```python
from build123d import *

# Parameters (mm, degrees)
SKETCH_1_W          = 18.46
SKETCH_1_H          = 19.3
EXTRUDE_1_DEPTH     = 1
CUT_EXTRUDE_1_DEPTH = 2


with BuildPart() as part:
    # 草图1 → 凸台-拉伸1 (new body)
    with BuildSketch(Plane(origin=(0, 0, 0), x_dir=(1, 0, 0), z_dir=(0, 1, 0))):
        Rectangle(SKETCH_1_W, SKETCH_1_H)
    extrude(amount=EXTRUDE_1_DEPTH)

    # 草图2 → 切除-拉伸1 (cut, through all)
    with BuildSketch(Plane(origin=(0, 1, 0), x_dir=(1, 0, 0), z_dir=(0, 1, 0))):
        with BuildLine():
            Line((9.23, -9.65), (8.03, -9.65))
            Line((8.03, -9.65), (8.03, -5.45))
            ThreePointArc((8.03, -5.45), (8.381471863, -4.601471863), (9.23, -4.25))
            Line((9.23, -4.25), (9.23, -9.65))
        make_face()
    extrude(amount=-CUT_EXTRUDE_1_DEPTH, mode=Mode.SUBTRACT)


solid = part.part
```
Can you work these out from the model? Positions are in its coordinate system, mm. A direction names the side the tool comes from. Give positions to 0.01 mm unless a question says otherwise; leave off trailing zeros. Write each loop counter-clockwise with the first axis right and the second up, starting at its lowest first coordinate (ties: lowest second). Pieces come first, ordered by that corner, then holes. Notation, with made-up numbers: (-34.5, 57.5) -> (-20.5, 57.5) arc R35 ccw to (-20.5, 91.5) -> close; hole circle Ø4 at (43, 83.25). An arc over 180 degrees is marked (long way). One line per item, written item: value.
Q1. Imagine slicing it at A-A on y = 0.75. Please give me the cut outline in (x, z).
Results found:
outline: (-9.23, -9.65) -> (9.23, -9.65) -> (9.23, 4.25) arc R1.2 cw to (8.03, 5.45) -> (8.03, 9.65) -> (-9.23, 9.65) -> close
Q2. Imagine slicing it at B-B on z = 4.5. Please give me the cut outline in (x, y), and give its area (3 significant figures).
Results found:
outline: (-9.23, 0) -> (8.5, 0) -> (8.5, 1) -> (-9.23, 1) -> close
area: 17.7 mm^2
Q3. Please list where these lines run through material, in increasing order: line 1 (X direction, y = 0.6, z = 6.25); line 2 (X direction, y = 0.85, z = 4.75). Write a range as [from, to].
Results found:
line 1: x = [-9.23, 8.03]
line 2: x = [-9.23, 8.26]
Q4. Which directions (+Z, -Z, +X, -X, +Y, -Y) give clear straight access to the entire face, cutting with the end or side of a thin tool? Please do faces 1 (the face through (-0.7, 0.5, 9.65)), 2 (the face through (8.03, 0.5, 7.6)).
Results found:
face 1: +Z, +X, -X, +Y, -Y
face 2: +Z, +X, +Y, -Y
